Build history of the part. All positions in model axes, mm. A direction names the side the tool comes from. Round coordinates to 2 decimals unless told otherwise and drop trailing zeros. Write each loop counter-clockwise with the first axis right and the second up, starting at its lowest first coordinate (ties: lowest second). Pieces come first, ordered by that corner, then holes.
from build123d import *

# Parameters (mm, degrees)
F0_W     = 4
F0_H     = 4
F1_DEPTH = 50
F3_DEPTH = 4
F5_DEPTH = 4


with BuildPart() as f1:
    # F0 (on Front) → F1 (new body)
    with BuildSketch(Plane.XZ):
        Rectangle(F0_W, F0_H)
    extrude(amount=F1_DEPTH)

    # F2 (on face) → F3 (cut)
    with BuildSketch(Plane(origin=(0, 0, 0), x_dir=(-1, 0, 0), z_dir=(0, 1, 0))):
        with BuildLine():
            ThreePointArc((-2, 0), (-1.4142135624, 1.4142135624), (0, 2))
            Line((0, 2), (-2, 2))
            Line((-2, 2), (-2, 0))
        make_face()
        with BuildLine():
            Line((-2, -2), (0, -2))
            ThreePointArc((0, -2), (-1.4142135624, -1.4142135624), (-2, 0))
            Line((-2, 0), (-2, -2))
        make_face()
        with BuildLine():
            Line((2, -2), (2, 0))
            ThreePointArc((2, 0), (1.4142135624, -1.4142135624), (0, -2))
            Line((0, -2), (2, -2))
        make_face()
        with BuildLine():
            ThreePointArc((0, 2), (1.4142135624, 1.4142135624), (2, 0))
            Line((2, 0), (2, 2))
            Line((2, 2), (0, 2))
        make_face()
    extrude(amount=-F3_DEPTH, mode=Mode.SUBTRACT)

    # F4 (on face) → F5 (cut)
    with BuildSketch(Plane.XZ.offset(50)):
        with BuildLine():
            ThreePointArc((-2, 0), (-1.4142135624, 1.4142135624), (0, 2))
            Line((0, 2), (-2, 2))
            Line((-2, 2), (-2, 0))
        make_face()
        with BuildLine():
            Line((-2, -2), (0, -2))
            ThreePointArc((0, -2), (-1.4142135624, -1.4142135624), (-2, 0))
            Line((-2, 0), (-2, -2))
        make_face()
        with BuildLine():
            Line((2, -2), (2, 0))
            ThreePointArc((2, 0), (1.4142135624, -1.4142135624), (0, -2))
            Line((0, -2), (2, -2))
        make_face()
        with BuildLine():
            ThreePointArc((0, 2), (1.4142135624, 1.4142135624), (2, 0))
            Line((2, 0), (2, 2))
            Line((2, 2), (0, 2))
        make_face()
    extrude(amount=-F5_DEPTH, mode=Mode.SUBTRACT)


solid = f1.part
1) Slice it at B-B (x = 1.3). Write the cut outline in (y, z).
Results:
outline: (-50, -1.52) - (-46, -1.52) - (-46, -2) - (-4, -2) - (-4, -1.52) - (0, -1.52) - (0, 1.52) - (-4, 1.52) - (-4, 2) - (-46, 2) - (-46, 1.52) - (-50, 1.52) - close
2) Slice it at A-A (z = -1.3). Write the cut outline in (x, y).
Results:
outline: (-2, -46) - (-1.52, -46) - (-1.52, -50) - (1.52, -50) - (1.52, -46) - (2, -46) - (2, -4) - (1.52, -4) - (1.52, 0) - (-1.52, 0) - (-1.52, -4) - (-2, -4) - close
3) Which spindle directions (+Z, -Z, +X, -X, +Y, -Y) get a long thin tool onto all of the face, cutting with end or side? Do faces 1 (the flat face through (1.6, -4, -1.5)), 2 (the flat face through (-1.5, -4, 1.6)), 3 (the flat face through (-1.6, -4, -1.6)). Say none if no direction does.
Results:
face 1: -Z, +X, +Y
face 2: +Z, -X, +Y
face 3: -Z, -X, +Y
4) Wall check: L1, parallel to Y at x = -1.7, z = -1.65; L2, parallel to Z at x = -1.5, y = -46.5; L3, parallel to Z at x = 1.8, y = -3. Give the ranges that are in metal, low to high.
Results:
L1: y = -46 to -4
L2: z = -1.32 to 1.32
L3: z = -0.87 to 0.87
5) Pin check, flat tip, straight feed: pin 1 Ø0.6 at (x, z) = (1, 1) entering from +Y. Stop position of the tip, or through.
Results:
pin 1: stops at y = 0
